Autodesk Inventor part; units mm, degrees
ref_plane "作業平面1" through (0, 0, -2.7) normal (0, 0, 1) x (1, 0, 0)
ref_plane "YZ Plane" through (0, 0, 0) normal (1, 0, 0) x (0, 1, 0)
ref_plane "XZ Plane" through (0, 0, 0) normal (0, 1, 0) x (-1, 0, 0)
sketch "スケッチ1" plane through (0, 0, 0) normal (0, 0, 1) x (1, 0, 0)
  line L0 (38, -55) -> (-38, -55)
  line L1 (-40, -53) -> (-40, 53)
  line L2 (-38, 55) -> (38, 55)
  line L3 (40, 53) -> (40, -53)
  line L4 (40, -55) -> (-40, 55) construction
  line L5 (-40, -55) -> (40, 55) construction
  line L6 (-38, 55) -> (-40, 53)
  line L7 (38, 55) -> (40, 53)
  line L8 (40, -53) -> (38, -55)
  line L9 (-38, -55) -> (-40, -53)
  circle A0 centre (-36, 51) radius 1.75
  line L10 (-56, 0) -> (56, 0) construction
  line L11 (0, -77) -> (0, 77) construction
  circle A1 centre (36, 51) radius 1.75
  circle A2 centre (-36, -51) radius 1.75
  circle A3 centre (36, -51) radius 1.75
  line L12 (31, -51) -> (-31, -51)
  line L13 (-36, -46) -> (-36, 46)
  line L14 (-31, 51) -> (31, 51)
  line L15 (36, 46) -> (36, -46)
  line L16 (36, -51) -> (-36, 51) construction
  line L17 (-36, -51) -> (36, 51) construction
  line L18 (-31, 51) -> (-36, 46)
  line L19 (36, 46) -> (31, 51)
  line L20 (-31, -51) -> (-36, -46)
  line L21 (31, -51) -> (36, -46)
  point P0 (0, 0)
  dimension "d1" = 80
  dimension "d2" = 110
  dimension "d3" = 2
  dimension "d4" = 2
  dimension "d5" = 2
  dimension "d6" = 2
  dimension "d7" = 2
  dimension "d8" = 2
  dimension "d9" = 2
  dimension "d10" = 2
  dimension "d11" = 3.5
  dimension "d12" = 4
  dimension "d13" = 4
  dimension "d14" = 4
  dimension "d15" = 4
  dimension "d16" = 5
  dimension "d17" = 5
  dimension "d18" = 5
  dimension "d19" = 5
  dimension "d20" = 5
  dimension "d21" = 5
  dimension "d22" = 5
  dimension "d23" = 5
extrude "押し出し1" add sketch "スケッチ1" against normal blind 30
ref_plane "作業平面1" through (0, 0, -2.7) normal (0, 0, 1) x (1, 0, 0)
sketch "スケッチ2" plane through (0, 0, -2.7) normal (0, 0, 1) x (1, 0, 0)
  line L0 (-56, 0) -> (56, 0) construction
  line L1 (0, -77) -> (0, 77) construction
  circle A0 centre (0, -15) radius 36 construction
  line L2 (31, -51) -> (-31, -51)
  circle A1 centre (0, -15) radius 30.5
  line L3 (-36, 20) -> (4, 20) construction
  line L4 (4, 20) -> (4, 36) construction
  line L5 (4, 36) -> (-36, 36) construction
  line L6 (-36, 36) -> (-36, 20) construction
  line L7 (-36, 20) -> (4, 36) construction
  line L8 (4, 20) -> (-36, 36) construction
  line L9 (-36, 46) -> (-31, 51) construction
  line L10 (-31, 51) -> (31, 51) construction
  line L11 (31, 51) -> (36, 46) construction
  line L12 (36, 46) -> (36, -46) construction
  line L13 (36, -46) -> (31, -51)
  line L14 (-31, -51) -> (-36, -46)
  line L15 (-36, -46) -> (-36, 46) construction
  circle A2 centre (25, 25) radius 12.5 construction
  circle A3 centre (0, -15) radius 34.5 construction
  line L16 (0, 19.5) -> (-36, 19.5)
  arc A4 (20.8327, 12.5) -> (0, 19.5) centre (0, -15) ccw
  line L17 (20.8327, 12.5) -> (31, 12.5)
  line L18 (-36, 19.5) -> (-36, -46)
  line L19 (36, 17.5) -> (36, -46)
  line L20 (31, 12.5) -> (36, 17.5)
  point P0 (0, 0)
  point P1 (-16, 28)
  point P2 (36, 12.5)
  dimension "d27" = 72
  dimension "d28" = 61
  dimension "d29" = 35
  dimension "d30" = 4
  dimension "d31" = 40
  dimension "d32" = 16
  dimension "d33" = 4
  dimension "d34" = 25
  dimension "d35" = 40
  dimension "d36" = 25
  dimension "d39" = 5
  dimension "d40" = 5
extrude "押し出し2" add sketch "スケッチ2" against normal up to surface (27.3 mm away)
sketch "スケッチ3" plane through (0, 0, -2.7) normal (0, 0, 1) x (1, 0, 0)
  line L0 (0, 19.5) -> (-36, 19.5)
  line L1 (-36, -46) -> (-36, 19.5)
  line L2 (-31, -51) -> (-36, -46)
  line L3 (31, -51) -> (-31, -51)
  line L4 (36, -46) -> (31, -51)
  line L5 (36, 17.5) -> (36, -46)
  line L6 (36, 17.5) -> (31, 12.5)
  line L7 (31, 12.5) -> (20.8327, 12.5)
  arc A0 (20.8327, 12.5) -> (0, 19.5) centre (0, -15) ccw
  circle A1 centre (0, -15) radius 30.5 construction
  circle A2 centre (0, -15) radius 33
  point P0 (0, 0)
  dimension "d41" = 66
extrude "押し出し3" add sketch "スケッチ3" along normal up to surface (2.7 mm away)
sketch "スケッチ4" plane through (0, 0, 0) normal (0, 0, 1) x (1, 0, 0)
  circle A0 centre (0, -15) radius 30.5 construction
  circle A1 centre (0, -15) radius 36 construction
  line L0 (0, -77) -> (0, 77) construction
  circle A2 centre (0, -51) radius 1.75
  circle A3 centre (31.1769, 3) radius 1.75
  circle A4 centre (-31.1769, 3) radius 1.75
  point P0 (0, 0)
  dimension "d44" = 72
  dimension "d45" = 3.5
  dimension "d48" = 360
extrude "押し出し4" cut sketch "スケッチ4" against normal through all
sketch "スケッチ5" plane through (0, 0, -30) normal (0, 0, -1) x (-1, 0, 0)
  circle A0 centre (-31.1769, 3) radius 1.75 construction
  circle A1 centre (31.1769, 3) radius 1.75 construction
  circle A2 centre (0, -51) radius 1.75 construction
  line L0 (-29.5603, 5.8) -> (-27.9438, 3)
  line L1 (-27.9438, 3) -> (-29.5603, 0.2)
  line L2 (-29.5603, 0.2) -> (-32.7935, 0.2)
  line L3 (-32.7935, 0.2) -> (-34.4101, 3)
  line L4 (-34.4101, 3) -> (-32.7935, 5.8)
  line L5 (-32.7935, 5.8) -> (-29.5603, 5.8)
  line L6 (32.7935, 5.8) -> (34.4101, 3)
  line L7 (34.4101, 3) -> (32.7935, 0.2)
  line L8 (32.7935, 0.2) -> (29.5603, 0.2)
  line L9 (29.5603, 0.2) -> (27.9438, 3)
  line L10 (27.9438, 3) -> (29.5603, 5.8)
  line L11 (29.5603, 5.8) -> (32.7935, 5.8)
  line L12 (1.6166, -48.2) -> (3.2332, -51)
  line L13 (3.2332, -51) -> (1.6166, -53.8)
  line L14 (1.6166, -53.8) -> (-1.6166, -53.8)
  line L15 (-1.6166, -53.8) -> (-3.2332, -51)
  line L16 (-3.2332, -51) -> (-1.6166, -48.2)
  line L17 (-1.6166, -48.2) -> (1.6166, -48.2)
  point P0 (0, 0)
  dimension "d52" = 5.6
extrude "押し出し5" cut sketch "スケッチ5" against normal blind 5
sketch "スケッチ6" plane through (0, 0, 0) normal (0, 1, 0) x (-1, 0, 0)
  line L0 (-4, -20) -> (4, -20)
  line L1 (4, -20) -> (4, -15)
  line L2 (4, -15) -> (-4, -15)
  line L3 (-4, -15) -> (-4, -20)
  line L4 (-4, -20) -> (4, -15) construction
  line L5 (4, -20) -> (-4, -15) construction
  line L6 (0, -62.7735) -> (0, 10.4622) construction
  line L7 (56, 0) -> (-56, 0) construction
  point P0 (0, 0)
  point P1 (0, -17.5)
  dimension "d55" = 5
  dimension "d56" = 8
  dimension "d57" = 17.5
extrude "押し出し6" cut sketch "スケッチ6" along normal up to surface (19.5 mm away)
chamfer "面取り1" distance 2 angle 45 4 edges at (-4, 17.3683, -20) (-4, 17.3683, -15) (4, 17.2519, -15) (4, 17.2519, -20)
equation "\"d4\" = d3"
equation "\"d5\" = d3"
equation "\"d6\" = d5"
equation "\"d7\" = d3"
equation "\"d8\" = d7"
equation "\"d9\" = d3"
equation "\"d10\" = d9"
equation "\"d17\" = d16"
equation "\"d19\" = d18"
equation "\"d20\" = d18"
equation "\"d21\" = d20"
equation "\"d22\" = d18"
equation "\"d23\" = d22"
properties part number "housing_3dp"
Can you work these out from the model? Positions are in its coordinate system, mm. A direction names the side the tool comes from. Coordinates: 2 decimals unless noted, no trailing zeros. Loops run counter-clockwise (first coordinate to the right, second up) from the corner with the lowest first, then second, coordinate; pieces in that order, holes last. Notation, with made-up numbers: (-6, 61.5) - (6, 61.5) arc R31 cw to (6, 86.5) - close; hole circle Ø8 at (-23.5, -5.75). An arc over 180 degrees is marked (long way). Put each result on its own line as item: value. Start each with the question number.
Item 1: If I drill on line 1 along Y through (x, z) = (0, -14.25); line 2 along X through (y, z) = (32.5, -2); line 3 along Y through (x, z) = (15, -13.75), over which ranges is the centre line in solid material (lowest first)?
Item 2: Suppose I cut it at A-A (y = -15). Please give me the cut outline in (x, z), and give its area (4 significant figures).
Item 3: If we mould it in two halves opening along Y, with no side actions, what happens to faces 1 (the face through (36, 32, -15)), 2 (the face through (-40, -1, -15)), 3 (the face through (1, -55, -15))? For each: +Y half, -Y half, draft (parallel to the pull), parting line (faces both ways), or undercut.
Item 4: Which directions (+Z, -Z, +X, -X, +Y, -Y) give clear straight access to the entire face, cutting with the end or side of a thin tool? Please do faces 4 (the face through (31, 0.2, -28)), 5 (the face through (-12, 17, 0)), 6 (the face through (0, 51, -15)).
Item 5: Suppose I cut it at B-B (z = -6.75). State how many separate pieces and enclosed holes the cut face has, and give its area (3 significant figures).
Item 6: Suppose I cut it at D-D (y = 14). Please give me the cut outline in (x, z), and give its area (3 significant figures).
Item 7: For pin 1 (4.5 mm diameter, centred on x = 32, y = 2.5, fed in from -Z); pin 2 (3 mm diameter, centred on x = -31.18, y = 3, fed in from -Z); pin 3 (3 mm diameter, centred on x = -32, y = 3.5, fed in from -Z), each with a flat end and sliding along its axis, tell me the tip position at first contact or that it passes through.
Item 8: Suppose I cut it at C-C (x = -25.5). Please give me the cut outline in (y, z).
Here are the results:
1. line 1: -55 to -52.75, -49.25 to -45.5, 15.5 to 19.5, 51 to 55
1. line 2: -40 to -36, 36 to 40
1. line 3: -55 to -41.56, 11.56 to 16.07, 51 to 55
2. outline: (-40, -30) - (-30.5, -30) - (-30.5, -2.7) - (-33, -2.7) - (-33, 0) - (-40, 0) - close; (30.5, -30) - (40, -30) - (40, 0) - (33, 0) - (33, -2.7) - (30.5, -2.7) - close
2. area: 556.5 mm²
3. face 1: undercut
3. face 2: draft
3. face 3: -Y half
4. face 4: -Z
4. face 5: +Z, +X, -X, +Y, -Y
4. face 6: +Z, -Z
5. separate pieces: 1
5. enclosed holes: 9
5. area: 3,420 mm²
6. outline: (-40, -30) - (-9.45, -30) - (-9.45, -2.7) - (-15.75, -2.7) - (-15.75, 0) - (-40, 0) - close; (9.45, -30) - (18.69, -30) - (18.69, 0) - (15.75, 0) - (15.75, -2.7) - (9.45, -2.7) - close; (32.5, -30) - (40, -30) - (40, 0) - (32.5, 0) - close
6. area: 1,380 mm²
7. pin 1: z = -30
7. pin 2: through
7. pin 3: z = -25
8. outline: (-55, -30) - (-31.73, -30) - (-31.73, -2.7) - (-35.95, -2.7) - (-35.95, 0) - (-55, 0) - close; (1.73, -30) - (19.5, -30) - (19.5, 0) - (5.95, 0) - (5.95, -2.7) - (1.73, -2.7) - close; (51, -30) - (55, -30) - (55, 0) - (51, 0) - close
